from build123d import *

# Parameters (mm, degrees)
SKETCH1_R           = 48
BOSS_EXTRUDE2_DEPTH = 10
SKETCH5_R           = 20
BOSS_EXTRUDE3_DEPTH = 30
SKETCH8_R           = 15
BOSS_EXTRUDE4_DEPTH = 30
SKETCH9_R           = 11.3
BOSS_EXTRUDE5_DEPTH = 45
SKETCH10_R          = 4
CUT_EXTRUDE1_DEPTH  = 45
FILLET1_R           = 10
CUT_EXTRUDE12_DEPTH = 21
SKETCH17_R          = 12.910346837
SKETCH17_R_2        = 9.35
CUT_EXTRUDE13_DEPTH = 2.5


with BuildPart() as part:
    # Sketch1 → Boss-Extrude2 (new body)
    with BuildSketch(Plane.XY):
        Circle(SKETCH1_R)
    extrude(amount=BOSS_EXTRUDE2_DEPTH)

    # Sketch5 → Boss-Extrude3 (add)
    with BuildSketch(Plane.XY):
        Circle(SKETCH5_R)
    extrude(amount=BOSS_EXTRUDE3_DEPTH)

    # Sketch8 → Boss-Extrude4 (add)
    with BuildSketch(Plane.XY.offset(30)):
        Circle(SKETCH8_R)
    extrude(amount=BOSS_EXTRUDE4_DEPTH)

    # Sketch9 → Boss-Extrude5 (add)
    with BuildSketch(Plane.XY.offset(60)):
        Circle(SKETCH9_R)
    extrude(amount=BOSS_EXTRUDE5_DEPTH)

    # Sketch10 → Cut-Extrude1 (cut)
    with BuildSketch(Plane.XY.offset(10)):
        with Locations((-37.5, 0)):
            Circle(SKETCH10_R)
        with Locations((-18.75, 32.475952642)):
            Circle(SKETCH10_R)
        with Locations((18.75, 32.475952642)):
            Circle(SKETCH10_R)
        with Locations((37.5, 0)):
            Circle(SKETCH10_R)
        with Locations((18.75, -32.475952642)):
            Circle(SKETCH10_R)
        with Locations((-18.75, -32.475952642)):
            Circle(SKETCH10_R)
    extrude(amount=-CUT_EXTRUDE1_DEPTH, mode=Mode.SUBTRACT)

    # Fillet1
    fillet1_edges = [part.edges().sort_by_distance(p)[0] for p in [
        (-20, 0, 10),
    ]]
    fillet(fillet1_edges, radius=FILLET1_R)

    # Sketch11 → Cut-Extrude12 (cut)
    with BuildSketch(Plane.XY.offset(105)):
        with BuildLine():
            Line((-10.377723879, 4.471336164), (-7.979912421, 4.901451086))
            ThreePointArc((-7.979912421, 4.901451086), (-7.707351037, 5.31977114), (-7.41288283, 5.722970658))
            Line((-7.41288283, 5.722970658), (-7.859673611, 8.118838016))
            ThreePointArc((-7.859673611, 8.118838016), (-9.29928676, 6.419755895), (-10.377723879, 4.471336164))
        make_face()
        with BuildLine():
            Line((-7.111084616, 8.781940309), (-4.788043642, 8.048469611))
            ThreePointArc((-4.788043642, 8.048469611), (-4.352299499, 8.292208034), (-3.904184691, 8.512377276))
            Line((-3.904184691, 8.512377276), (-3.186383203, 10.841446494))
            ThreePointArc((-3.186383203, 10.841446494), (-5.250700172, 10.006005582), (-7.111084616, 8.781940309))
        make_face()
        with BuildLine():
            Line((-2.215381565, 11.080707763), (-0.499291766, 9.351680744))
            ThreePointArc((-0.499291766, 9.351680744), (-0.000188596, 9.364999998), (0.498915109, 9.351700846))
            Line((0.498915109, 9.351700846), (2.216869197, 11.080410234))
            ThreePointArc((2.216869197, 11.080410234), (0.000758547, 11.299999975), (-2.215381565, 11.080707763))
        make_face()
        with BuildLine():
            ThreePointArc((3.903841837, 8.512534518), (4.351965512, 8.292383324), (4.787719471, 8.048662452))
            Line((4.787719471, 8.048662452), (7.112263581, 8.780985523))
            ThreePointArc((7.112263581, 8.780985523), (5.252043492, 10.005300553), (3.187838704, 10.841018605))
            Line((3.187838704, 10.841018605), (3.903841837, 8.512534518))
        make_face()
        with BuildLine():
            ThreePointArc((7.412652321, 5.723269221), (7.707136768, 5.320081564), (7.979715, 4.901772487))
            Line((7.979715, 4.901772487), (10.37832409, 4.469942851))
            ThreePointArc((10.37832409, 4.469942851), (9.300148567, 6.418507352), (7.860763544, 8.117782733))
            Line((7.860763544, 8.117782733), (7.412652321, 5.723269221))
        make_face()
        with BuildLine():
            ThreePointArc((9.22331349, 1.622871918), (9.296695871, 1.129013232), (9.343653989, 0.631945518))
            Line((9.343653989, 0.631945518), (11.266835622, -0.865109859))
            ThreePointArc((11.266835622, -0.865109859), (11.291705862, -0.432872656), (11.3, 0))
            ThreePointArc((11.3, 0), (11.157319766, 1.790032301), (10.732882188, 3.534860667))
            Line((10.732882188, 3.534860667), (9.22331349, 1.622871918))
        make_face()
        with BuildLine():
            ThreePointArc((8.921024692, -2.849305783), (8.756493988, -3.320698426), (8.567074452, -3.782652553))
            Line((8.567074452, -3.782652553), (9.574250893, -6.001976327))
            ThreePointArc((9.574250893, -6.001976327), (10.565414534, -4.007744468), (11.146226868, -1.857855378))
            Line((11.146226868, -1.857855378), (8.921024692, -2.849305783))
        make_face()
        with BuildLine():
            ThreePointArc((6.575036647, -6.668741867), (6.210284859, -7.009678093), (5.827881402, -7.33069051))
            Line((5.827881402, -7.33069051), (5.688320667, -9.76386235))
            ThreePointArc((5.688320667, -9.76386235), (7.492718241, -8.458674445), (9.006105299, -6.824959145))
            Line((9.006105299, -6.824959145), (6.575036647, -6.668741867))
        make_face()
        with BuildLine():
            ThreePointArc((2.722786944, -8.960449557), (2.241374312, -9.092824984), (1.753590957, -9.199355616))
            Line((1.753590957, -9.199355616), (0.499264728, -11.288965175))
            ThreePointArc((0.499264728, -11.288965175), (2.703530495, -10.971824044), (4.802793542, -10.228547023))
            Line((4.802793542, -10.228547023), (2.722786944, -8.960449557))
        make_face()
        with BuildLine():
            ThreePointArc((-4.804166743, -10.227902126), (-2.705003505, -10.97146098), (-0.500780336, -11.288898044))
            Line((-0.500780336, -11.288898044), (-1.753220435, -9.199426238))
            ThreePointArc((-1.753220435, -9.199426238), (-2.24100808, -9.092915252), (-2.722426043, -8.960559215))
            Line((-2.722426043, -8.960559215), (-4.804166743, -10.227902126))
        make_face()
        with BuildLine():
            Line((-5.689631474, -9.76309857), (-5.827586141, -7.330925233))
            ThreePointArc((-5.827586141, -7.330925233), (-6.210002527, -7.009928218), (-6.574768046, -6.669006683))
            Line((-6.574768046, -6.669006683), (-9.007021511, -6.823749959))
            ThreePointArc((-9.007021511, -6.823749959), (-7.493853802, -8.457668426), (-5.689631474, -9.76309857))
        make_face()
        with BuildLine():
            Line((-9.575056609, -6.000690871), (-8.566922092, -3.782997605))
            ThreePointArc((-8.566922092, -3.782997605), (-8.756360234, -3.321051107), (-8.920909924, -2.849665091))
            Line((-8.920909924, -2.849665091), (-11.146476196, -1.856358912))
            ThreePointArc((-11.146476196, -1.856358912), (-10.565952503, -4.006325961), (-9.575056609, -6.000690871))
        make_face()
        with BuildLine():
            Line((-11.266951667, -0.86359721), (-9.343679434, 0.631569185))
            ThreePointArc((-9.343679434, 0.631569185), (-9.296741337, 1.128638789), (-9.223378847, 1.622500431))
            Line((-9.223378847, 1.622500431), (-10.732407515, 3.53630159))
            ThreePointArc((-10.732407515, 3.53630159), (-11.217518819, 1.3628175), (-11.266951667, -0.86359721))
        make_face()
    extrude(amount=-CUT_EXTRUDE12_DEPTH, mode=Mode.SUBTRACT)

    # Sketch17 → Cut-Extrude13 (cut)
    with BuildSketch(Plane(origin=(0, 0, 100), x_dir=(-1, 0, 0), z_dir=(0, 0, -1))):
        Circle(SKETCH17_R)
        Circle(SKETCH17_R_2, mode=Mode.SUBTRACT)
    extrude(amount=-CUT_EXTRUDE13_DEPTH, mode=Mode.SUBTRACT)


solid = part.part
Check sheet for the modelled part. Datum: model origin and axes. Units: mm. A direction names the side the tool comes from. Give positions to 0.01 mm unless a question says otherwise; leave off trailing zeros. Write each loop counter-clockwise with the first axis right and the second up, starting at its lowest first coordinate (ties: lowest second). Pieces come first, ordered by that corner, then holes. Notation, with made-up numbers: M 15.5,-13 L 39.5,-13 A30 ccw 39.5,17 Z; hole C 61,72.5 d6. An arc over 180 degrees is marked long. Use one line per item in the form item = value.
(1) Section check C-C on z = 61.5. Record the boundary of the cut face in (x, y), plus the area to 3 significant figures.
Answer block:
outline = C 0,0 d22.6
area = 401 mm2
(2) Section check A-A on x = 40. Record the boundary of the cut face in (y, z), plus the area to 3 significant figures.
Answer block:
outline = M -26.53,0 L -3.12,0 L -3.12,10 L -26.53,10 Z; M 3.12,0 L 26.53,0 L 26.53,10 L 3.12,10 Z
area = 468 mm2
(3) Tool access check on faces 1 (the cylindrical face through (-4.336, -19.524, 24.93)), 2 (the flat face through (5, 9, 84)). Record the directions out of +Z, -Z, +X, -X, +Y, -Y that give a thin tool (end or side, any length) a straight path to the whole face; none if there is none.
Answer block:
face_1 = +Z
face_2 = +Z, +Y
(4) Material ranges on line 1 along Y through (x, z) = (18, 3); line 2 along Y through (x, z) = (-18.75, 4); line 3 along Y through (x, z) = (37, 7), recorded low to high.
Answer block:
line_1 = -44.5 to -36.41, -28.55 to 28.55, 36.41 to 44.5
line_2 = -44.19 to -36.48, -28.48 to 28.48, 36.48 to 44.19
line_3 = -30.58 to -3.97, 3.97 to 30.58
(5) Section check B-B on y = -34. Record the boundary of the cut face in (x, z).
Answer block:
outline = M -33.88,0 L -22.45,0 L -22.45,10 L -33.88,10 Z; M -15.05,0 L 15.05,0 L 15.05,10 L -15.05,10 Z; M 22.45,0 L 33.88,0 L 33.88,10 L 22.45,10 Z
(6) Depth check by flat-ended pin: P1, Ø2, axis at x = -15.5, y = -5, coming from the +Z side; P2, Ø4, axis at x = 17, y = -7.5, coming from the -Z side; P3, Ø13, axis at x = -37.5, y = 0, coming from the +Z side; P4, Ø0.8, axis at x = -9.5, y = -4.5, coming from the +Z side. Enter the tip coordinate at first touch or a pass-through.
Answer block:
P1 = 30
P2 = 0
P3 = 10
P4 = 84
(7) Draft check along X on faces 3 (the flat face through (-22, -21, 10)), 4 (the cylindrical face through (-40.7, -2.4, 5.1)), 5 (the cylindrical face through (2.027, -9.128, 101.232)). Enter one of: pulls with the +X half, pulls with the -X half, needs draft (parallel to the pull), parting line crosses it, or undercut.
Answer block:
face_3 = needs draft
face_4 = undercut
face_5 = parting line crosses it
(8) Section check D-D on x = -37.5. Record the boundary of the cut face in (y, z).
Answer block:
outline = M -29.96,0 L -4,0 L -4,10 L -29.96,10 Z; M 4,0 L 29.96,0 L 29.96,10 L 4,10 Z
